The listing builds one solid part. Answer for the finished solid, in the listing's coordinates (mm). Face numbers are marked on the shaded views. Round coordinates to 2 decimals unless told otherwise and drop trailing zeros. Loops run counter-clockwise (first coordinate to the right, second up) from the corner with the lowest first, then second, coordinate; pieces in that order, holes last. Notation, with made-up numbers: M 23.25,-38.5 L 55.25,-38.5 A19 ccw 55.25,-21.5 Z; hole C 49,26.25 d5. An arc over 180 degrees is marked long. Answer as a JSON object with one key per item and string values.
```python
from build123d import *

# Parameters (mm, degrees)
EXTRUDE_1_DEPTH     = 10
SKETCH_2_R          = 1.25
CUT_EXTRUDE_1_DEPTH = 64.188882811
SKETCH_3_W          = 16
SKETCH_3_H          = 2
CUT_EXTRUDE_2_DEPTH = 10


with BuildPart() as part:
    # Эскиз1 → Бобышка-Вытянуть1 (new body)
    with BuildSketch(Plane(origin=(0, 0, 0), x_dir=(1, 0, 0), z_dir=(0, 1, 0))):
        with BuildLine():
            Line((-28.118262676, 42.740270437), (-27.170876932, 54.566519955))
            Line((-27.170876932, 54.566519955), (-29.023121545, 54.714900905))
            Line((-29.023121545, 54.714900905), (-29.972465165, 42.864211138))
            ThreePointArc((-29.972465165, 42.864211138), (-29.243677502, 40.224761685), (-26.987939543, 38.672514561))
            ThreePointArc((-26.987939543, 38.672514561), (-15.177415755, 32.289756522), (-7.695453225, 21.143083968))
            Line((-7.695453225, 21.143083968), (0, 0))
            Line((0, 0), (1.879385242, 0.684040287))
            Line((1.879385242, 0.684040287), (-5.816067983, 21.827124254))
            ThreePointArc((-5.816067983, 21.827124254), (-13.882439346, 33.815300424), (-26.617286688, 40.642186829))
            ThreePointArc((-26.617286688, 40.642186829), (-27.751256034, 41.416884799), (-28.118262676, 42.740270437))
        make_face()
    extrude(amount=EXTRUDE_1_DEPTH)

    # Эскиз2 → Вырез-Вытянуть1 (cut, through all)
    with BuildSketch(Plane(origin=(0, 0, 0), x_dir=(0, 0, -1), z_dir=(1, 0, 0))):
        with Locations((48.653395196, 5)):
            Circle(SKETCH_2_R)
    extrude(amount=-CUT_EXTRUDE_1_DEPTH, mode=Mode.SUBTRACT)

    # Эскиз3 → Вырез-Вытянуть2 (cut)
    with BuildSketch(Plane(origin=(1.879385242, 0, -0.684040287), x_dir=(-0.34202014332566943, 0, -0.9396926207859082), z_dir=(0.9396926207859082, 0, -0.34202014332566943))):
        with Locations((11.25, 5)):
            Rectangle(SKETCH_3_W, SKETCH_3_H)
    extrude(amount=-CUT_EXTRUDE_2_DEPTH, mode=Mode.SUBTRACT)


solid = part.part
```
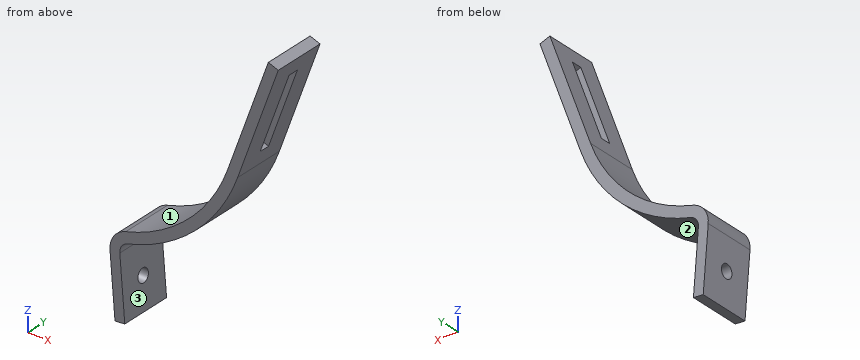
Item 1: Determine the mould class of the marked faces 1, 2 and 3 for opening direction Z: released by +Z, released by -Z, zero draft, split by the parting line, or undercut.
Values follow:
{"face 1": "released by +Z", "face 2": "released by -Z", "face 3": "undercut"}
Item 2: Straight lines are drawn through the part: line 1 (Z direction, x = -28.7, y = 5); line 2 (X direction, y = 7.5, z = -51.5); line 3 (X direction, y = 3.75, z = -15.5). For each, find the intervals that lie inside material, in ascending order.
Values follow:
{"line 1": "-54.69 to -49.9, -47.4 to -39.61", "line 2": "-29.28 to -27.42", "line 3": "-5.64 to -3.51"}
Item 3: The part is cut by section B-B (z = -4.5). Give the vertices of the cut face in (x, y).
Values follow:
{"outline": "M -1.64,0 L 0.49,0 L 0.49,4 L -1.64,4 Z; M -1.64,6 L 0.49,6 L 0.49,10 L -1.64,10 Z"}
Item 4: The part is cut by section D-D (y = 1.25). Give the vertices of the cut face in (x, z), then the cut area to 3 significant figures.
Values follow:
{"outline": "M -29.97,-42.86 L -29.02,-54.71 L -27.17,-54.57 L -28.12,-42.74 A2 cw -26.62,-40.64 A30 ccw -5.82,-21.83 L 1.88,-0.68 L 0,0 L -7.7,-21.14 A28 cw -26.99,-38.67 A4 ccw Z", "area": "131 mm^2"}
Item 5: The part is cut by section A-A (y = 5). Give the vertices of the cut face in (x, z).
Values follow:
{"outline": "M -29.97,-42.86 L -29.61,-47.4 L -27.74,-47.4 L -28.12,-42.74 A2 cw -26.62,-40.64 A30 ccw -5.82,-21.83 L -4.7,-18.77 L -6.58,-18.09 L -7.7,-21.14 A28 cw -26.99,-38.67 A4 ccw Z; M -29.41,-49.9 L -29.02,-54.71 L -27.17,-54.57 L -27.54,-49.9 Z; M -1.11,-3.05 L 0.77,-3.74 L 1.88,-0.68 L 0,0 Z"}
Item 6: The part is cut by section C-C (x = -4). Give the vertices of the cut face in (y, z).
Values follow:
{"outline": "M 0,-16.84 L 4,-16.84 L 4,-10.99 L 0,-10.99 Z; M 6,-16.84 L 10,-16.84 L 10,-10.99 L 6,-10.99 Z"}
Item 7: Flat-ended cylindrical pins translate along their axes: P1, Ø4, axis at x = -18, y = 3.5, coming from the +Z side; P2, Ø1, axis at y = 6, z = -36, coming from the +X side; P3, Ø3, axis at y = 5, z = -48.65, coming from the -X side. Find the tip coordinate at first contact, or state that the pin passes through.
Values follow:
{"P1": "z = -33.01", "P2": "x = -15.92", "P3": "x = -29.63"}
